Part model, mm, in its own coordinate system. A direction names the side the tool comes from. Give positions to 0.01 mm unless a question says otherwise; leave off trailing zeros. Write each loop counter-clockwise with the first axis right and the second up, starting at its lowest first coordinate (ties: lowest second). Pieces come first, ordered by that corner, then holes. Notation, with made-up numbers: M 59.5,73 L 108.5,73 A12 cw 108.5,96 Z; hole C 3.5,20 d3. An arc over 180 degrees is marked long. Answer as CSV lines item,"result". Start each with the question number.
1) Wall check: line 1 along Y through (x, z) = (0, 42); line 2 along Z through (x, y) = (1, -19.5); line 3 along Y through (x, z) = (-19, 2.95). Give the ranges that are in metal, low to high. Write a range as from..to.
2) Tool access for faces 4 (the flat face through (0, 14, 41)), 5 (the flat face through (0, 19, 4)): list every direction of +Z, -Z, +X, -X, +Y, -Y with a clear straight run to the whole face (end or side of a thin tool).
3) Slice it at A-A, the plane y = 24.5. Give the cut face in (x, z), plus the area to 3 significant figures.
4) Pin check, flat tips, straight feed: pin 1 Ø8 at (x, z) = (7.5, 33) entering from -Y; pin 2 Ø12 at (x, z) = (13, 7.5) entering from -Y; pin 3 Ø2 at (x, y) = (-19, 0) entering from -Z. Stop position of each tip, or through.
5) Slice it at D-D, the plane y = 13.5. Give the cut face in (x, z).
6) Mould opens along Y. For faces 1 (the cylindrical face through (-0.26, -10.167, 43.535)), 2 (the cylindrical face through (0.27, -20.22, 1.97)), 3 (the cylindrical face through (-25.865, 10.724, 22.185)) say: pulls with the +Y half, pulls with the -Y half, needs draft (parallel to the pull), parting line crosses it, or undercut.
7) Slice it at B-B, the plane x = -14.5. Give the cut face in (y, z), plus the area to 3 significant figures.
8) Slice it at C-C, the plane z = 22.5. Give the cut face in (x, y), plus the area to 3 significant figures.
```python
from build123d import *

# Parameters (mm, degrees)
SKETCH_1_R          = 28
EXTRUDE_1_DEPTH     = 45
SKETCH_2_R          = 1.25
CUT_EXTRUDE_1_DEPTH = 4
SKETCH_3_R          = 1.25
CUT_EXTRUDE_2_DEPTH = 5
SKETCH_4_R          = 21.25
EXTRUDE_2_DEPTH     = 1
SKETCH_5_R          = 1.5
CUT_EXTRUDE_3_DEPTH = 5
SKETCH_6_R          = 2
CUT_EXTRUDE_4_DEPTH = 5


with BuildPart() as part:
    # 草图1 → 凸台-拉伸1 (new body)
    with BuildSketch(Plane.XY):
        with Locations(Location((0, 0, 0), (0, 0, 180))):
            Circle(SKETCH_1_R)
    extrude(amount=EXTRUDE_1_DEPTH)

    # 草图2 → 切除-拉伸1 (cut)
    with BuildSketch(Plane(origin=(0, 0, 0), x_dir=(-1, 0, 0), z_dir=(0, 0, -1))):
        with Locations((19, 0)):
            Circle(SKETCH_2_R)
        with Locations((0, -19)):
            Circle(SKETCH_2_R)
        with Locations((-19, 0)):
            Circle(SKETCH_2_R)
        with Locations((0, 19)):
            Circle(SKETCH_2_R)
    extrude(amount=-CUT_EXTRUDE_1_DEPTH, mode=Mode.SUBTRACT)

    # 草图3 → 切除-拉伸2 (cut)
    with BuildSketch(Plane.XY.offset(45)):
        with Locations((0, 24.5)):
            Circle(SKETCH_3_R)
        with Locations((21.217622393, -12.25)):
            Circle(SKETCH_3_R)
        with Locations((-21.217622393, -12.25)):
            Circle(SKETCH_3_R)
    extrude(amount=-CUT_EXTRUDE_2_DEPTH, mode=Mode.SUBTRACT)

    # 草图4 → 凸台-拉伸2 (add)
    with BuildSketch(Plane.XY.offset(45)):
        Circle(SKETCH_4_R)
    extrude(amount=EXTRUDE_2_DEPTH)

    # 草图5 → 切除-拉伸3 (cut)
    with BuildSketch(Plane.XY.offset(46)):
        with Locations((0, 13.5)):
            Circle(SKETCH_5_R)
        with Locations((11.691342951, -6.75)):
            Circle(SKETCH_5_R)
        with Locations((-11.691342951, -6.75)):
            Circle(SKETCH_5_R)
    extrude(amount=-CUT_EXTRUDE_3_DEPTH, mode=Mode.SUBTRACT)

    # 草图6 → 切除-拉伸4 (cut)
    with BuildSketch(Plane.XY.offset(46)):
        with Locations((0, -12.15)):
            Circle(SKETCH_6_R)
        with Locations((-10.522208656, 6.075)):
            Circle(SKETCH_6_R)
        with Locations((10.522208656, 6.075)):
            Circle(SKETCH_6_R)
    extrude(amount=-CUT_EXTRUDE_4_DEPTH, mode=Mode.SUBTRACT)


solid = part.part
```
Found:
1,line 1,"-28..-14.15, -10.15..12, 15..23.25, 25.75..28"
1,line 2,"4..46"
1,line 3,"-20.57..-1.25, 1.25..20.57"
2,face 4,"+Z"
2,face 5,"-Z"
3,outline,"M -13.56,0 L 13.56,0 L 13.56,45 L 1.25,45 L 1.25,40 L -1.25,40 L -1.25,45 L -13.56,45 Z"
3,area,"1,210 mm²"
4,pin 1,"y = -27.78"
4,pin 2,"y = -27.11"
4,pin 3,"z = 4"
5,outline,"M -24.53,0 L 24.53,0 L 24.53,45 L 16.41,45 L 16.41,46 L 1.5,46 L 1.5,41 L -1.5,41 L -1.5,46 L -16.41,46 L -16.41,45 L -24.53,45 Z"
6,face 1,"undercut"
6,face 2,"undercut"
6,face 3,"parting line crosses it"
7,outline,"M -23.95,0 L 23.95,0 L 23.95,45 L 15.53,45 L 15.53,46 L -15.53,46 L -15.53,45 L -23.95,45 Z"
7,area,"2,190 mm²"
8,outline,"C 0,0 d56"
8,area,"2,460 mm²"
